```python
from build123d import *

# Parameters (mm, degrees)
SKETCH1_R           = 4.7625
SKETCH1_R_2         = 12.7
BOSS_EXTRUDE1_DEPTH = 3.175
SCALE1_SCALE        = 0.6


with BuildPart() as part:
    # Sketch1 → Boss-Extrude1 (new body)
    with BuildSketch(Plane(origin=(0, 0, 0), x_dir=(1, 0, 0), z_dir=(0, 1, 0))):
        with BuildLine():
            Line((0, -8.73125), (-23.925972084, -8.73125))
            ThreePointArc((-23.925972084, -8.73125), (-31.985998621, -11.616670426), (-36.383573946, -18.961805556))
            ThreePointArc((-36.383573946, -18.961805556), (-62.075355484, -28.106340634), (-57.903987761, -1.156575296))
            Line((-57.903987761, -1.156575296), (-27.611137885, 11.086197953))
            ThreePointArc((-27.611137885, 11.086197953), (-24.427259651, 9.943349405), (-25.202507899, 6.650603808))
            Line((-25.202507899, 6.650603808), (-30.057631482, 3.251009676))
            ThreePointArc((-30.057631482, 3.251009676), (-31.032259676, -2.276381482), (-25.504868518, -3.251009676))
            Line((-25.504868518, -3.251009676), (-9.212459777, 8.157057741))
            ThreePointArc((-9.212459777, 8.157057741), (-8.346095505, 8.584301319), (-7.391354591, 8.73125))
            Line((-7.391354591, 8.73125), (0, 8.73125))
            ThreePointArc((0, 8.73125), (8.73125, 0), (0, -8.73125))
        make_face()
        with Locations(Location((0, 0, 0), (0, 0, 270))):
            Circle(SKETCH1_R, mode=Mode.SUBTRACT)
        with Locations(Location((-51.955576272, -15.875, 0), (0, 0, 270))):
            Circle(SKETCH1_R_2, mode=Mode.SUBTRACT)
    extrude(amount=BOSS_EXTRUDE1_DEPTH)


with BuildPart() as part_1:
    # Scale1: scaled about (-29.432275391, 1.5875, 5.297099312)
    add(part.part.scale(SCALE1_SCALE).moved(Location((-11.772910156, 0.635, 2.118839725))))


solid = part_1.part
```
Part model, mm, in its own coordinate system. A direction names the side the tool comes from. Coordinates: 2 decimals unless noted, no trailing zeros. Write each loop counter-clockwise with the first axis right and the second up, starting at its lowest first coordinate (ties: lowest second). Pieces come first, ordered by that corner, then holes.
Item 1: Slice it at D-D (x = -15.5). Write the cut outline in (y, z) (3 decimals), and give its area (3 significant figures).
Item 2: Probe line 1 (X direction, y = 1.85, z = 4.75); line 2 (X direction, y = 0.95, z = 1.5); line 3 (Z direction, x = -42.5, y = 2.05). List the from-to ranges inside material, lowest first.
Item 3: Mould opens along X. For faces 5 (the face through (-14.308, 1.574, 3.437)), 6 (the face through (-6.535, 1.574, 2.004)), 7 (the face through (-29, 2.54, 5)) say: released by +X, released by -X, zero draft, split by the parting line, or undercut.
Item 4: Slice it at C-C (y = 1.3). Count the separate pieces of the cut face and the enclosed holes in it, and give its area (3 significant figures).
Item 5: Which spindle directions (+Z, -Z, +X, -X, +Y, -Y) get a long thin tool onto all of the face, cutting with end or side? Do faces 1 (the face through (-16.79, 1.57, -3.03)), 2 (the face through (-28.331, 1.574, -0.866)), 3 (the face through (-19, 2, 7.358)), 4 (the face through (-14, 2, -3.12)). Say none if no direction does.
Item 6: Slice it at B-B (z = 10.5). Write the cut outline in (x, y) (3 decimals), and give its area (3 significant figures).
Item 7: Pin check, flat tips, straight feed: pin 1 (1 mm diameter, centred on y = 1, z = 5, fed in from -X); pin 2 (3.5 mm diameter, centred on x = -11.77, z = 2.12, fed in from -Y); pin 3 (3 mm diameter, centred on x = -39.5, z = -1.5, fed in from -Y) (3 decimals). Stop position of each tip, or through.
Item 8: Slice it at A-A (x = -41.5). Write the cut outline in (y, z) (3 decimals).
Results found:
1. outline: (0.635, -3.12) - (2.54, -3.12) - (2.54, 7.358) - (0.635, 7.358) - close
1. area: 20.0 mm2
2. line 1: x = -49.52 to -46.19, -39.7 to -12.89, -10.66 to -7.24
2. line 2: x = -43.27 to -30.74, -23.41 to -14.56, -8.98 to -6.57
2. line 3: z = 1.19 to 4.04, 19.25 to 21.16
3. face 5: undercut
3. face 6: released by +X
3. face 7: zero draft
4. separate pieces: 1
4. enclosed holes: 2
4. area: 355 mm2
5. face 1: -Z, +Y, -Y
5. face 2: +Y, -Y
5. face 3: +Z, +X, +Y, -Y
5. face 4: -Z, +X, +Y, -Y
6. outline: (-52.402, 0.635) - (-50.48, 0.635) - (-50.48, 2.54) - (-52.402, 2.54) - close; (-35.413, 0.635) - (-32.294, 0.635) - (-32.294, 2.54) - (-35.413, 2.54) - close
6. area: 9.60 mm2
7. pin 1: stops at x = -50.22
7. pin 2: passes through
7. pin 3: stops at y = 0.635
8. outline: (0.635, 0.786) - (2.54, 0.786) - (2.54, 4.162) - (0.635, 4.162) - close; (0.635, 19.125) - (2.54, 19.125) - (2.54, 21.058) - (0.635, 21.058) - close
